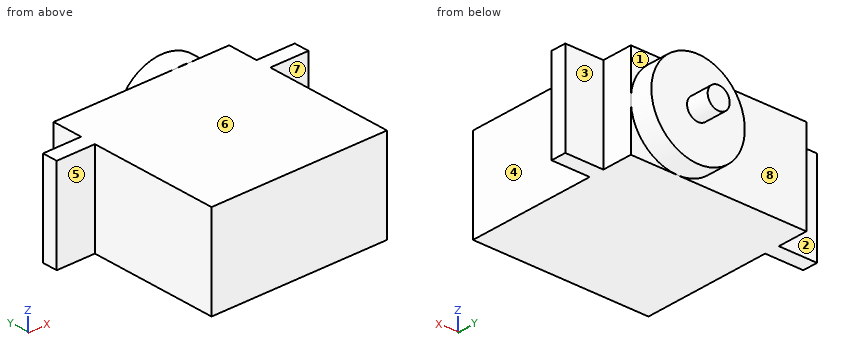
```python
from build123d import *

# Parameters (mm, degrees)
BOSS_EXTRUDE1_DEPTH = 12.2
SKETCH2_R           = 6.126682997
BOSS_EXTRUDE2_DEPTH = 3
SKETCH3_R           = 1.445
BOSS_EXTRUDE3_DEPTH = 3


with BuildPart() as part:
    # Sketch1 → Boss-Extrude1 (new body)
    with BuildSketch(Plane.XY):
        Polygon((0, 0), (23, 0), (23, 17), (28, 17), (28, 19), (23, 19), (23, 23), (0, 23), (0, 19), (-5, 19), (-5, 17), (0, 17), align=None)
    extrude(amount=BOSS_EXTRUDE1_DEPTH)

    # Sketch2 → Boss-Extrude2 (add)
    with BuildSketch(Plane(origin=(0, 23, 0), x_dir=(1, 0, 0), z_dir=(0, 1, 0))):
        with Locations((16.884532498, -6.126394767)):
            Circle(SKETCH2_R)
    extrude(amount=BOSS_EXTRUDE2_DEPTH)

    # Sketch3 → Boss-Extrude3 (add)
    with BuildSketch(Plane(origin=(0, 26, 0), x_dir=(1, 0, 0), z_dir=(0, 1, 0))):
        with Locations((16.884532498, -6.126394767)):
            Circle(SKETCH3_R)
    extrude(amount=BOSS_EXTRUDE3_DEPTH)


solid = part.part
```
Check sheet for the modelled part. Datum: model origin and axes. Units: mm. Face numbers are marked on the shaded views. A direction names the side the tool comes from. Coordinates: 2 decimals unless noted, no trailing zeros. Order: outer loops, then holes, each group sorted by start corner. A loop starts at its lowest first (then second) coordinate and runs counter-clockwise, first axis right, second up. Notation, with made-up numbers: (0, -15) -> (37, -15) arc R20 ccw to (37, -3) -> close; hole circle Ø9 at (32.5, 22.25). An arc over 180 degrees is marked (long way). Write item = value, one per line. Start each with the question number.
1) Cross-section at B-B (x = 2.5). Enter the section's corners in (y, z).
2) Material ranges on L1, parallel to X at y = 2, z = 5.5; L2, parallel to Z at x = 7.5, y = 6.75; L3, parallel to X at y = 23.25, z = 6, recorded low to high.
3) Mould release check, pull along Y, two halves, no side actions. Record for the marked faces 6, 7 and 8: +Y half, -Y half, draft (parallel to the pull), parting line (faces both ways), or undercut.
4) Go/stop test with flat-tipped pins: P1, Ø2.5, axis at x = -3.5, z = 7, coming from the +Y side; P2, Ø2, axis at x = 1.5, z = 3.5, coming from the +Y side; P3, Ø1.5, axis at x = 24.5, y = 20.5, coming from the -Z side; P4, Ø4, axis at x = -2.5, z = 9, coming from the -Y side. Record where each tip stops, or that it passes through.
5) Access from +Z, -Z, +X, -X, +Y, -Y to the whole of each face (thin tool, end or side, straight path). Record for the marked faces 1, 2, 3, 4 and 5.
6) Cross-section at A-A (z = 1). Enter the section's corners in (x, y).
7) Cross-section at D-D (z = 2.75). Enter the section's corners in (x, y), then the cut area to 3 significant figures.
Ans:
q1.outline = (0, 0) -> (23, 0) -> (23, 12.2) -> (0, 12.2) -> close
q2.L1 = 0 to 23
q2.L2 = 0 to 12.2
q2.L3 = 10.76 to 23.01
q3.face_6 = draft
q3.face_7 = -Y half
q3.face_8 = +Y half
q4.P1 = 19
q4.P2 = 23
q4.P3 = through
q4.P4 = 17
q5.face_1 = +Z, +X, +Y
q5.face_2 = +Z, -Z, -X, +Y
q5.face_3 = +Z, -Z, +X, +Y
q5.face_4 = +Z, -Z, +X, -Y
q5.face_5 = +Z, -Z, -X, -Y
q6.outline = (-5, 17) -> (0, 17) -> (0, 0) -> (23, 0) -> (23, 17) -> (28, 17) -> (28, 19) -> (23, 19) -> (23, 23) -> (20.24, 23) -> (20.24, 26) -> (13.53, 26) -> (13.53, 23) -> (0, 23) -> (0, 19) -> (-5, 19) -> close
q7.outline = (-5, 17) -> (0, 17) -> (0, 0) -> (23, 0) -> (23, 17) -> (28, 17) -> (28, 19) -> (23, 19) -> (23, 23) -> (22, 23) -> (22, 26) -> (11.77, 26) -> (11.77, 23) -> (0, 23) -> (0, 19) -> (-5, 19) -> close
q7.area = 580 mm²
